```python
from build123d import *

# Parameters (mm, degrees)
SKETCH2_W                = 250
SKETCH2_H                = 250
BOSS_EXTRUDE1_DEPTH      = 250
SKETCH3_W                = 210
SKETCH3_H                = 200
CUT_EXTRUDE1_DEPTH       = 220
BOSS_EXTRUDE2_REACH      = 363.974
FILLET1_R                = 100
FILLET2_R                = 20
SKETCH11_R               = 60
CUT_EXTRUDE2_DEPTH       = 344.693177122
SKETCH12_W               = 250
SKETCH12_H               = 10
BOSS_EXTRUDE3_DEPTH      = 90
BOSS_EXTRUDE4_START      = 20
SKETCH13_W               = 5
SKETCH13_H               = 20
BOSS_EXTRUDE4_DEPTH      = 50
BOSS_EXTRUDE5_START      = 20
SKETCH14_W               = 5
SKETCH14_H               = 42
BOSS_EXTRUDE5_DEPTH      = 50
SKETCH15_W               = 20
SKETCH15_H               = 40
CUT_EXTRUDE3_DEPTH       = 20
SKETCH17_W               = 20
SKETCH17_H               = 40
CUT_EXTRUDE5_DEPTH       = 23
SKETCH18_W               = 20
SKETCH18_H               = 10
BOSS_EXTRUDE6_DEPTH      = 20
SKETCH19_W               = 250
SKETCH19_H               = 50
CUT_EXTRUDE11_DEPTH      = 70
SKETCH24_W               = 200
SKETCH24_H               = 95
CUT_EXTRUDE12_DEPTH      = 70
CUT_EXTRUDE14_DEPTH      = 414.793426724
SKETCH26_W               = 75
SKETCH26_H               = 50
CUT_EXTRUDE15_DEPTH      = 344.693177122
BOSS_EXTRUDE7_REACH      = 415.793
SKETCH27_W               = 50
SKETCH27_H               = 25
CUT_EXTRUDE16_DEPTH      = 374.296129099
CUT_EXTRUDE16_DEPTH_BACK = 374.296129099
SKETCH28_W               = 50
SKETCH28_H               = 25
FILLET3_R                = 10
SKETCH29_W               = 20
SKETCH29_H               = 39.615
BOSS_EXTRUDE8_DEPTH      = 95


with BuildPart() as part:
    # Sketch2 → Boss-Extrude1 (new body)
    with BuildSketch(Plane(origin=(0, 0, 0), x_dir=(1, 0, 0), z_dir=(0, 1, 0))):
        Rectangle(SKETCH2_W, SKETCH2_H)
    extrude(amount=BOSS_EXTRUDE1_DEPTH)

    # Sketch3 → Cut-Extrude1 (cut)
    with BuildSketch(Plane(origin=(0, 250, 0), x_dir=(1, 0, 0), z_dir=(0, 1, 0))):
        with Locations((0, -25)):
            Rectangle(SKETCH3_W, SKETCH3_H)
    extrude(amount=-CUT_EXTRUDE1_DEPTH, mode=Mode.SUBTRACT)

    # Sketch5 → Boss-Extrude2 (add, up to next)
    with BuildSketch(Plane.ZY.offset(-105), mode=Mode.PRIVATE) as boss_extrude2_sk1:
        Polygon((125, 30), (125, 80), (-75, 30), align=None)
    boss_extrude2_tool1 = extrude(boss_extrude2_sk1.sketch, amount=BOSS_EXTRUDE2_REACH, mode=Mode.PRIVATE) - part.part
    add(boss_extrude2_tool1.solids().sort_by_distance((105, 46.666667, 58.333333))[0])

    # Fillet1
    fillet1_edges = [part.edges().sort_by_distance(p)[0] for p in [
        (-105, 55, 25),
        (105, 55, 25),
    ]]
    fillet(fillet1_edges, radius=FILLET1_R)

    # Fillet2
    fillet2_edges = [part.edges().sort_by_distance(p)[0] for p in [
        (115, 250, 125),
        (-115, 250, 125),
        (105, 250, 25),
        (0, 250, -75),
        (-105, 250, 25),
    ]]
    fillet(fillet2_edges, radius=FILLET2_R - 0.0001)  # a hair under: the kernel refuses the full size

    # Sketch11 → Cut-Extrude2 (cut, through all)
    with BuildSketch(Plane.XY.offset(-75)):
        with Locations((0, 130)):
            Circle(SKETCH11_R)
    extrude(amount=-CUT_EXTRUDE2_DEPTH, mode=Mode.SUBTRACT)

    # Sketch12 → Boss-Extrude3 (add)
    with BuildSketch(Plane(origin=(0, 0, -125), x_dir=(-1, 0, 0), z_dir=(0, 0, -1))):
        with Locations((0, 5)):
            Rectangle(SKETCH12_W, SKETCH12_H)
    extrude(amount=BOSS_EXTRUDE3_DEPTH)

    # Sketch13 → Boss-Extrude4 (add)
    with BuildSketch(Plane(origin=(0, 0, -125), x_dir=(-1, 0, 0), z_dir=(0, 0, -1)).offset(BOSS_EXTRUDE4_START)):
        Polygon((-70, 35), (-70, 30), (-65, 30), (0, 30), (0, 35), align=None)
        Polygon((0, 35), (0, 30), (65, 30), (70, 30), (70, 35), align=None)
        with Locations((67.5, 20)):
            Rectangle(SKETCH13_W, SKETCH13_H)
        with Locations((-67.5, 20)):
            Rectangle(SKETCH13_W, SKETCH13_H)
    extrude(amount=BOSS_EXTRUDE4_DEPTH)

    # Sketch14 → Boss-Extrude5 (add)
    with BuildSketch(Plane(origin=(0, 0, -125), x_dir=(-1, 0, 0), z_dir=(0, 0, -1)).offset(BOSS_EXTRUDE5_START)):
        with Locations((24.5, 56)):
            Rectangle(SKETCH14_W, SKETCH14_H)
        with Locations((-24.5, 56)):
            Rectangle(SKETCH14_W, SKETCH14_H)
    extrude(amount=BOSS_EXTRUDE5_DEPTH)

    # Sketch15 → Cut-Extrude3 (cut)
    with BuildSketch(Plane(origin=(125, 0, 0), x_dir=(0, 0, -1), z_dir=(1, 0, 0))):
        with Locations((54.23, 147.66)):
            Rectangle(SKETCH15_W, SKETCH15_H)
    extrude(amount=-CUT_EXTRUDE3_DEPTH, mode=Mode.SUBTRACT)

    # Sketch17 → Cut-Extrude5 (cut)
    with BuildSketch(Plane(origin=(125, 0, 0), x_dir=(0, 0, -1), z_dir=(1, 0, 0))):
        with Locations((54.23, 142.66)):
            Rectangle(SKETCH17_W, SKETCH17_H)
    extrude(amount=-CUT_EXTRUDE5_DEPTH, mode=Mode.SUBTRACT)

    # Sketch18 → Boss-Extrude6 (add)
    with BuildSketch(Plane(origin=(125, 0, 0), x_dir=(0, 0, -1), z_dir=(1, 0, 0))):
        with Locations((54.23, 162.66)):
            Rectangle(SKETCH18_W, SKETCH18_H)
    extrude(amount=-BOSS_EXTRUDE6_DEPTH)

    # Sketch19 → Cut-Extrude11 (cut)
    with BuildSketch(Plane.ZY.offset(125)):
        with Locations((0, 225)):
            Rectangle(SKETCH19_W, SKETCH19_H)
    extrude(amount=-CUT_EXTRUDE11_DEPTH, mode=Mode.SUBTRACT)

    # Sketch24 → Cut-Extrude12 (cut)
    with BuildSketch(Plane.ZY.offset(125)):
        with Locations((25, 152.5)):
            Rectangle(SKETCH24_W, SKETCH24_H)
    extrude(amount=-CUT_EXTRUDE12_DEPTH, mode=Mode.SUBTRACT)

    # Sketch25 → Cut-Extrude14 (cut, through all)
    with BuildSketch(Plane.ZY.offset(125)):
        Polygon((125, 105), (-30, 105), (-30, 200), (-75, 200), (-75, 250), (125, 250), align=None)
    extrude(amount=-CUT_EXTRUDE14_DEPTH, mode=Mode.SUBTRACT)

    # Sketch26 → Cut-Extrude15 (cut, through all)
    with BuildSketch(Plane.XY.offset(-75)):
        with Locations((87.5, 225)):
            Rectangle(SKETCH26_W, SKETCH26_H)
    extrude(amount=-CUT_EXTRUDE15_DEPTH, mode=Mode.SUBTRACT)

    # Boss-Extrude7: up to this face of the body (flat: up to its plane)
    boss_extrude7_end = Plane(part.part.faces().sort_by_distance((-125, 66.05015674, -19.686520376))[0])
    # Sketch27 → Boss-Extrude7 (add, up to the picked face)
    with BuildSketch(Plane(origin=(125, 0, 0), x_dir=(0, 0, -1), z_dir=(1, 0, 0)), mode=Mode.PRIVATE) as boss_extrude7_sk1:
        with Locations((100, 212.5)):
            Rectangle(SKETCH27_W, SKETCH27_H)
    boss_extrude7_tool1 = split(extrude(boss_extrude7_sk1.sketch, amount=-BOSS_EXTRUDE7_REACH, mode=Mode.PRIVATE), bisect_by=boss_extrude7_end, keep=Keep.BOTH, mode=Mode.PRIVATE)
    add(boss_extrude7_tool1.solids().sort_by(Axis((125, 212.5, -100), (-1, 0, 0)))[0])

    # Sketch28 → Cut-Extrude16 (cut, two sides: drawn at the far end of the back side and taken through both)
    with BuildSketch(Plane(origin=(50, 0, 0), x_dir=(0, 0, -1), z_dir=(1, 0, 0)).offset(-CUT_EXTRUDE16_DEPTH_BACK)):
        with Locations((100, 237.5)):
            Rectangle(SKETCH28_W, SKETCH28_H)
    extrude(amount=CUT_EXTRUDE16_DEPTH + CUT_EXTRUDE16_DEPTH_BACK, mode=Mode.SUBTRACT)

    # Fillet3
    fillet3_edges = [part.edges().sort_by_distance(p)[0] for p in [
        (-125, 165, -75),
        (-125, 105, 25),
        (125, 225, -100),
        (125, 212.5, -75),
        (-125, 225, -100),
    ]]
    fillet(fillet3_edges, radius=FILLET3_R)

    # Sketch29 → Boss-Extrude8 (add)
    with BuildSketch(Plane(origin=(0, 200, 0), x_dir=(1, 0, 0), z_dir=(0, 1, 0))):
        with Locations((115, 49.8075)):
            Rectangle(SKETCH29_W, SKETCH29_H)
    extrude(amount=-BOSS_EXTRUDE8_DEPTH)


solid = part.part
```
Model file for the job. Use its own axes, mm. A direction names the side the tool comes from. Give positions to 0.01 mm unless a question says otherwise; leave off trailing zeros. Loops run counter-clockwise (first coordinate to the right, second up) from the corner with the lowest first, then second, coordinate; pieces in that order, holes last. Notation, with made-up numbers: (-32, 65.25) - (26, 65.25) arc R32 ccw to (26, 99.25) - close; hole circle Ø5 at (29.5, 10.25). An arc over 180 degrees is marked (long way). One line per item, written item: value. Start each with the question number.
1. Slice it at A-A (x = 0). List the corners of the cut face in (y, z).
2. Pull direction X, two halves, no side cores. Call faces 1 (the flat face through (-27, 56, -170)), 2 (the flat face through (103, 105, 66)), 3 (the flat face through (0, 35, -170)): pulls with the +X half, pulls with the -X half, needs draft (parallel to the pull), parting line crosses it, or undercut.
3. Slice it at B-B (z = -183.5). List the corners of the cut face in (x, y), plus the area to 3 significant figures.
4. Slice it at C-C (y = 163). List the corners of the cut face in (x, z), plus the area to 3 significant figures.
5. Probe L1, parallel to X at y = 130, z = -100; L2, parallel to Y at x = -3, z = -136.5; L3, parallel to Z at x = 104, y = 78. List the from-to ranges inside material, lowest first. Write a range as from..to.
6. Which spindle directions (+Z, -Z, +X, -X, +Y, -Y) get a long thin tool onto all of the face, cutting with end or side? Do faces 4 (the flat face through (48, 35, -170)), 5 (the flat face through (-103, 105, 46)), 6 (the cylindrical face through (61.45, 72.31, 22.27)). Say none if no direction does.
7. Pin check, flat tips, straight feed: pin 1 (16 mm diameter, centred on y = 19, z = -166.5, fed in from +X); pin 2 (22 mm diameter, centred on x = -6, z = -168.5, fed in from +Y); pin 3 (1 mm diameter, centred on x = 68, y = 160.5, fed in from +Z). Stop position of each tip, or through.
8. Slice it at D-D (z = -113). List the corners of the cut face in (x, y), plus the area to 3 significant figures.
Solution:
1. outline: (0, -215) - (10, -215) - (10, -125) - (70, -125) - (70, -75) - (30, -75) - (80, 125) - (0, 125) - close; (30, -195) - (35, -195) - (35, -145) - (30, -145) - close; (190, -125) - (225, -125) - (225, -75) - (190, -75) - close
2. face 1: pulls with the -X half
2. face 2: needs draft
2. face 3: undercut
3. outline: (-125, 0) - (125, 0) - (125, 10) - (70, 10) - (70, 35) - (27, 35) - (27, 77) - (22, 77) - (22, 35) - (-22, 35) - (-22, 77) - (-27, 77) - (-27, 35) - (-70, 35) - (-70, 10) - (-125, 10) - close; hole (-65, 10) - (65, 10) - (65, 30) - (-65, 30) - close
3. area: 3,820 mm^2
4. outline: (-125, -125) - (-50.11, -125) - (-50.11, -75) - (-115, -75) arc R10 ccw to (-125, -85) - close; (50.11, -125) - (125, -125) - (125, -30) - (105, -30) - (105, -75) - (50.11, -75) - close
4. area: 8,370 mm^2
5. L1: x = -125..-60, 60..125
5. L2: y = 0..10
5. L3: z = -125..125
6. face 4: -Z, +X, +Y
6. face 5: +Z, -X, +Y
6. face 6: +Y
7. pin 1: stops at x = 70
7. pin 2: stops at y = 35
7. pin 3: stops at z = -75
8. outline: (-125, 0) - (125, 0) - (125, 215) arc R10 ccw to (115, 225) - (-115, 225) arc R10 ccw to (-125, 215) - close; hole circle Ø120 at (0, 130)
8. area: 44,900 mm^2
